Can you work these out from the drawing? Everything is in mm from the part's minimum corner. A direction names the side the tool comes from. Round coordinates to 2 decimals unless told otherwise and drop trailing zeros. Loops run counter-clockwise (first coordinate to the right, second up) from the corner with the lowest first, then second, coordinate; pieces in that order, holes last. Notation, with made-up numbers: (6, -27.75) -> (22, -27.75) arc R33 cw to (22, 9.25) -> close; hole circle Ø10 at (6.25, -2). An arc over 180 degrees is marked (long way). One line per item, written item: value.
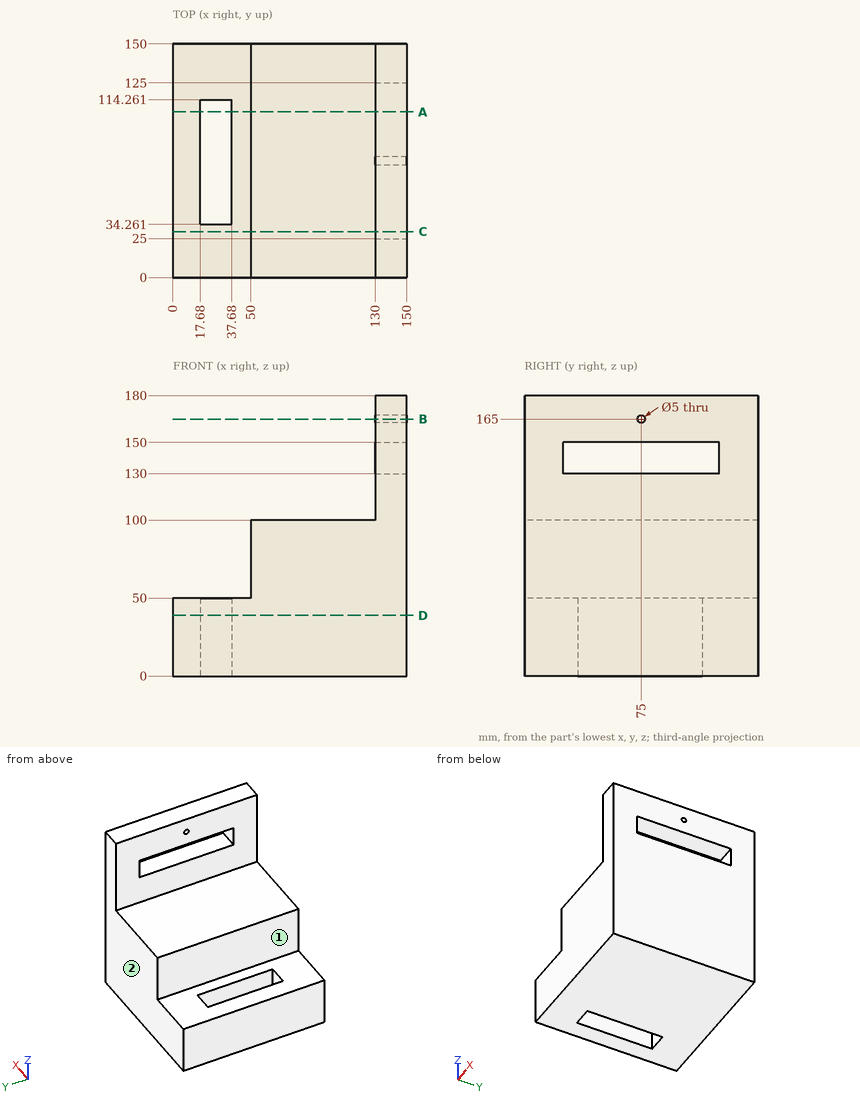
(1) If we section it at C-C, the plane y = 29.5: Please give me the cut outline in (x, z), then the cut area to 3 significant figures.
Recorded:
outline: (0, 0) -> (150, 0) -> (150, 130) -> (130, 130) -> (130, 100) -> (50, 100) -> (50, 50) -> (0, 50) -> close; (130, 150) -> (150, 150) -> (150, 180) -> (130, 180) -> close
area: 13,700 mm²
(2) If we section it at B-B, the plane z = 165: Please give me the cut outline in (x, y), then the cut area to 3 significant figures.
Recorded:
outline: (130, 0) -> (150, 0) -> (150, 72.5) -> (130, 72.5) -> close; (130, 77.5) -> (150, 77.5) -> (150, 150) -> (130, 150) -> close
area: 2,900 mm²
(3) If we section it at A-A, the plane y = 106.5: Please give me the cut outline in (x, z).
Recorded:
outline: (0, 0) -> (17.68, 0) -> (17.68, 50) -> (0, 50) -> close; (37.68, 0) -> (150, 0) -> (150, 130) -> (130, 130) -> (130, 100) -> (50, 100) -> (50, 50) -> (37.68, 50) -> close; (130, 150) -> (150, 150) -> (150, 180) -> (130, 180) -> close
(4) For the marked faces 1 and 2, which set-ups out of +Z, -Z, +X, -X, +Y, -Y let a thin tool reach every point of the face, with its end or its side?
Recorded:
face 1: +Z, -X, +Y, -Y
face 2: +Z, -Z, +X, -X, +Y
(5) If we section it at D-D, the plane z = 39: Please give me the cut outline in (x, y).
Recorded:
outline: (0, 0) -> (150, 0) -> (150, 150) -> (0, 150) -> close; hole (17.68, 34.26) -> (37.68, 34.26) -> (37.68, 114.26) -> (17.68, 114.26) -> close
(6) I'm going to push flat-ended pins straight in: pin 1 Ø24 at (y, z) = (79, 144) entering from -X; pin 2 Ø15 at (x, y) = (26, 107) entering from +Z; pin 3 Ø2 at (x, z) = (128.5, 139.5) entering from -Y; pin 4 Ø5 at (x, y) = (72, 109) entering from +Z. Where does each tip first touch, or does it pass through?
Recorded:
pin 1: x = 130
pin 2: z = 50
pin 3: through
pin 4: z = 100
(7) If I drill on L1, parallel to Z at x = 145.5, y = 75; L2, parallel to Y at x = 142, z = 165; L3, parallel to X at y = 78, z = 23.5, over which ranges is the centre line in solid material (lowest first)?
Recorded:
L1: 0 to 130, 150 to 162.5, 167.5 to 180
L2: 0 to 72.5, 77.5 to 150
L3: 0 to 17.68, 37.68 to 150
